Here's how the part is built. I have some questions about the finished solid (model axes, mm). A direction names the side the tool comes from. Round coordinates to 2 decimals unless told otherwise and drop trailing zeros. Order: outer loops, then holes, each group sorted by start corner. A loop starts at its lowest first (then second) coordinate and runs counter-clockwise, first axis right, second up. Notation, with made-up numbers: M -4.5,13 L 25.5,13 A31 ccw 25.5,49 Z; hole C 68.25,-0.5 d5. An arc over 180 degrees is marked long. Write item = value, one per line. Start each with the question number.
Item 1: I'm going to push flat-ended pins straight in: P1, Ø5, axis at y = -99.5, z = 145.5, coming from the -X side; P2, Ø12, axis at y = 52.5, z = 162, coming from the -X side; P3, Ø1, axis at x = -111.5, y = 27, coming from the +Z side; P4, Ø8, axis at x = 85.5, y = 84, coming from the -Z side. Where does each tip first touch, or does it pass through?
Item 2: For faces 1 (the face through (-37.302, -167.983, 39.589)), 2 (the face through (-19.527, 148.724, 152.962)), 3 (the face through (-2, 2, 2.5)), which set-ups out of +Z, -Z, +X, -X, +Y, -Y let a thin tool reach every point of the face, with its end or its side?
Item 3: I want a section at D-D, the plane z = 35.5. List the corners of the cut face in (x, y) for me, plus the area to 3 significant figures.
Item 4: We'd pull the mould along Z, two halves only. Please class faces 4 (the face through (-2, 2, 0)), 5 (the face through (112, -101, 210)), 6 (the face through (151.028, -10.492, 123.304)): pulls with the +Z half, pulls with the -Z half, needs draft (parallel to the pull), parting line crosses it, or undercut.
Item 5: I want a section at C-C, the plane z = 120. List the corners of the cut face in (x, y) for me.
Item 6: I want a section at A-A, the plane x = 0. List the corners of the cut face in (y, z) for me.
Item 7: Please list where these lines run through material, in increasing order: L1, parallel to Z at x = 150.3, y = 0; L2, parallel to Y at x = 0, z = 169; L3, parallel to Z at x = -157.5, y = 35.5.
Item 8: I want a section at B-B, the plane z = 145.5. List the corners of the cut face in (x, y) for me.
```python
from build123d import *

# Parameters (mm, degrees)
F0_R     = 170
F1_DEPTH = 100
F1_TAPER = -3
F7_R     = 152.5
F2_DEPTH = 110
F4_T     = -2.5
F6_D     = 22
F6_DEPTH = 200
F6_START = 47.8972388
F6_TIP   = 6.6094668093


with BuildPart() as f1:
    # F0 (on Top) → F1 (new body)
    with BuildSketch(Plane.XY):
        Circle(F0_R)
    extrude(amount=F1_DEPTH, taper=F1_TAPER)

    # F7 (on face) → F2 (join)
    with BuildSketch(Plane.XY.offset(100)):
        Circle(F7_R)
    extrude(amount=F2_DEPTH)

    # F4
    f4_openings = [f1.faces().sort_by_distance(p)[0] for p in [
        (0, 0, 210),
    ]]
    offset(amount=F4_T, openings=f4_openings, kind=Kind.INTERSECTION)

    # F6
    # its depths count from where the whole tool has entered the part; down to there all is cleared
    with Locations(Plane.YZ.offset(200).offset(-F6_START)):
        with Locations((0, 120)):
            Hole(F6_D / 2, depth=F6_DEPTH)
            with Locations((0, 0, -(F6_DEPTH + F6_TIP / 2))):  # 118° drill point
                Cone(0, F6_D / 2, F6_TIP, mode=Mode.SUBTRACT)


solid = f1.part
```
Filled in:
q1.P1 = -117.67
q1.P2 = -145.24
q1.P3 = 2.5
q1.P4 = 0
q2.face_1 = -Z
q2.face_2 = +Z
q2.face_3 = none
q3.outline = C 0,0 d343.72; hole C 0,0 d338.71
q3.area = 2,680 mm^2
q4.face_4 = pulls with the -Z half
q4.face_5 = pulls with the +Z half
q4.face_6 = undercut
q5.outline = M 149.6,-11 A150 cw long 149.6,11 L 152.1,11 A152.5 ccw long 152.1,-11 Z
q6.outline = M -175.24,100 L -170,0 L 170,0 L 175.24,100 L 152.5,100 L 152.5,210 L 150,210 L 150,97.5 L 172.61,97.5 L 167.63,2.5 L -167.63,2.5 L -172.61,97.5 L -150,97.5 L -150,210 L -152.5,210 L -152.5,100 Z
q7.L1 = 0 to 2.5, 97.5 to 109, 131 to 210
q7.L2 = -152.5 to -150, 150 to 152.5
q7.L3 = 0 to 2.5, 97.5 to 100
q8.outline = C 0,0 d305; hole C 0,0 d300
